Answer from the drawing. Dimensions are ordinates in mm from the lowest x, y and z of the part. Coordinates: 2 decimals unless noted, no trailing zeros. Write each loop counter-clockwise with the first axis right and the second up, starting at its lowest first coordinate (ties: lowest second). Pieces come first, ordered by that corner, then holes.
(1) Given P1, Ø1.9, axis at x = 64.95, z = 41.2, coming from the -Y side, flat-ended and moving along its own axis, determine where the tip first touches the part or whether it passes through.
(2) The part is cut by section A-A on z = 3.7. Determine the outline of the cut face in (x, y).
(3) Straight lines are drawn through the part: line 1 (Z direction, x = 64.95, y = 6.75); line 2 (X direction, y = 3, z = 41.2). For each, find the intervals that lie inside material, in ascending order.
(4) The part is cut by section B-B on x = 3.45. Determine the outline of the cut face in (y, z), plus the area to 3 significant figures.
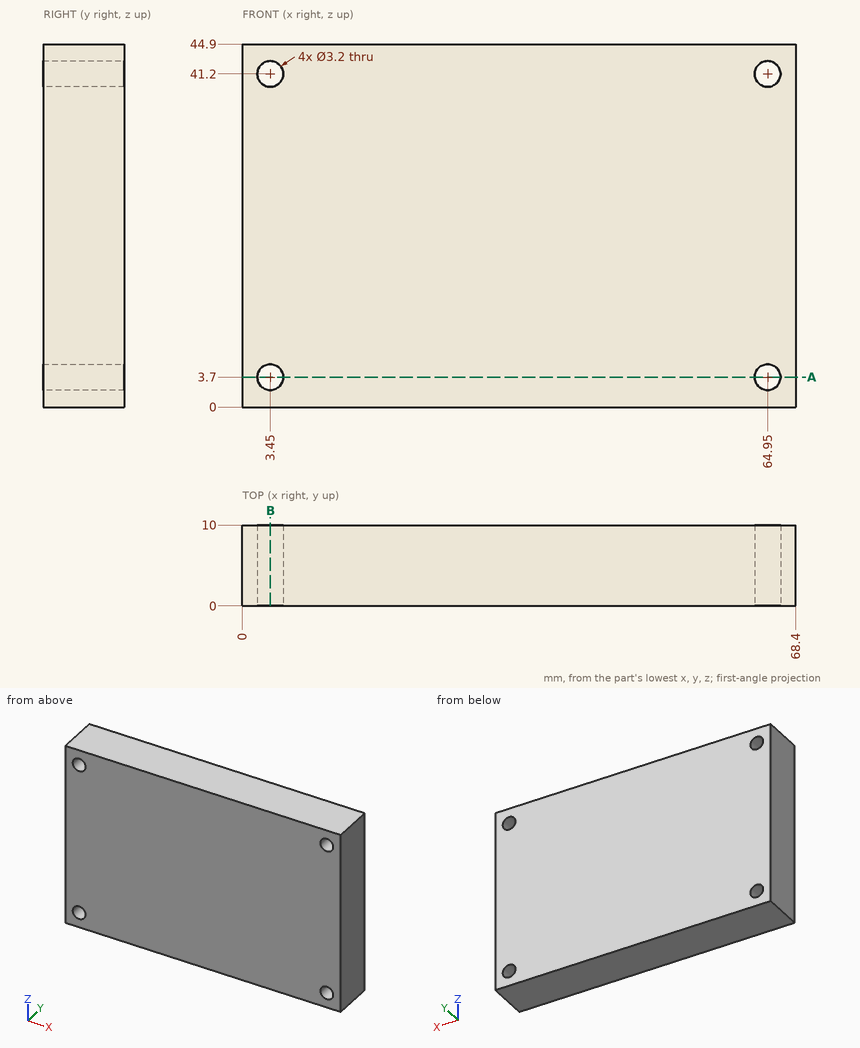
Model answer:
1. P1: passes through
2. outline: (0, 0) - (1.85, 0) - (1.85, 10) - (0, 10) - close; (5.05, 0) - (63.35, 0) - (63.35, 10) - (5.05, 10) - close; (66.55, 0) - (68.4, 0) - (68.4, 10) - (66.55, 10) - close
3. line 1: z = 0 to 2.1, 5.3 to 39.6, 42.8 to 44.9
3. line 2: x = 0 to 1.85, 5.05 to 63.35, 66.55 to 68.4
4. outline: (0, 0) - (10, 0) - (10, 2.1) - (0, 2.1) - close; (0, 5.3) - (10, 5.3) - (10, 39.6) - (0, 39.6) - close; (0, 42.8) - (10, 42.8) - (10, 44.9) - (0, 44.9) - close
4. area: 385 mm2
